```python
from build123d import *

# Parameters (mm, degrees)
ESBO_O1_W                  = 115.09677689
ESBO_O1_H                  = 63
RESSALTO_EXTRUS_O1_DEPTH   = 2
FILETE1_R                  = 3
CORTE_EXTRUS_O4_DEPTH      = 66.635866816
CORTE_EXTRUS_O4_DEPTH_BACK = 66.635866816
ESBO_O6_W                  = 7
ESBO_O6_H                  = 9
ESBO_O7_R                  = 1.5
CORTE_EXTRUS_O5_DEPTH      = 66.635866816


with BuildPart() as part:
    # Esboço1 → Ressalto-extrusão1 (new body)
    with BuildSketch(Plane(origin=(0, 0, 0), x_dir=(1, 0, 0), z_dir=(0, 1, 0))):
        Rectangle(ESBO_O1_W, ESBO_O1_H)
    extrude(amount=RESSALTO_EXTRUS_O1_DEPTH)

    # Filete1
    filete1_edges = [part.edges().sort_by_distance(p)[0] for p in [
        (-57.548388445, 1, -31.5),
        (57.548388445, 1, -31.5),
        (57.548388445, 1, 31.5),
        (-57.548388445, 1, 31.5),
    ]]
    fillet(filete1_edges, radius=FILETE1_R)

    # Esboço6 → Corte-extrusão4 (cut, two sides: drawn at the far end of the back side and taken through both)
    with BuildSketch(Plane(origin=(0, 2, 0), x_dir=(1, 0, 0), z_dir=(0, 1, 0)).offset(-CORTE_EXTRUS_O4_DEPTH_BACK)):
        with Locations((-39.048388445, 0)):
            Rectangle(ESBO_O6_W, ESBO_O6_H)
        with Locations((39.048388445, 0)):
            Rectangle(ESBO_O6_W, ESBO_O6_H)
    extrude(amount=CORTE_EXTRUS_O4_DEPTH + CORTE_EXTRUS_O4_DEPTH_BACK, mode=Mode.SUBTRACT)

    # Esboço7 → Corte-extrusão5 (cut, through all)
    with BuildSketch(Plane(origin=(0, 2, 0), x_dir=(1, 0, 0), z_dir=(0, 1, 0))):
        with Locations(Location((-45.998388445, 27.5, 0), (0, 0, 270))):
            Circle(ESBO_O7_R)
        with Locations(Location((45.998388445, 27.5, 0), (0, 0, 90))):
            Circle(ESBO_O7_R)
        with Locations(Location((45.998388445, -27.5, 0), (0, 0, 270))):
            Circle(ESBO_O7_R)
        with Locations(Location((-45.998388445, -27.5, 0), (0, 0, 90))):
            Circle(ESBO_O7_R)
    extrude(amount=-CORTE_EXTRUS_O5_DEPTH, mode=Mode.SUBTRACT)


solid = part.part
```
For this review, take the finished solid that the model builds, in its own axes (mm). A direction names the side the tool comes from. Coordinates: 2 decimals unless noted, no trailing zeros. Write each loop counter-clockwise with the first axis right and the second up, starting at its lowest first coordinate (ties: lowest second). Pieces come first, ordered by that corner, then holes.
(1) Tool access review of faces 1 (the face through (-1, 0, 0)), 2 (the face through (-42.548, 1, 0)): name each direction out of +Z, -Z, +X, -X, +Y, -Y from which nothing blocks a thin tool from reaching the whole face with its end or side.
(2) For pin 1 Ø2.5 at (x, z) = (46, -27.5) entering from +Y, flat-tipped, find the tip position at first contact; note if it passes through.
(3) Add section A-A on y = 0.35. Give the boundary of the cut face in (x, z).
(4) Wall thickness on probe 1 along X at (y, z) = (0.9, -2); probe 2 along X at (y, z) = (1.4, -27.5); probe 3 along Z at (x, y) = (-45, 1.65): over which ranges is each line inside the solid? List them lowest first.
Answer sheet:
1. face 1: +Z, -Z, +X, -X, -Y
1. face 2: +Y, -Y
2. pin 1: passes through
3. outline: (-57.55, -28.5) arc R3 ccw to (-54.55, -31.5) - (54.55, -31.5) arc R3 ccw to (57.55, -28.5) - (57.55, 28.5) arc R3 ccw to (54.55, 31.5) - (-54.55, 31.5) arc R3 ccw to (-57.55, 28.5) - close; hole circle Ø3 at (-46, -27.5); hole circle Ø3 at (-46, 27.5); hole (-42.55, -4.5) - (-35.55, -4.5) - (-35.55, 4.5) - (-42.55, 4.5) - close; hole (35.55, -4.5) - (42.55, -4.5) - (42.55, 4.5) - (35.55, 4.5) - close; hole circle Ø3 at (46, -27.5); hole circle Ø3 at (46, 27.5)
4. probe 1: x = -57.55 to -42.55, -35.55 to 35.55, 42.55 to 57.55
4. probe 2: x = -57.55 to -47.5, -44.5 to 44.5, 47.5 to 57.55
4. probe 3: z = -31.5 to -28.62, -26.38 to 26.38, 28.62 to 31.5
